Geometry: final body of the model. Coordinates: model frame, mm. Face numbers are marked on the shaded views. A direction names the side the tool comes from. Coordinates: 2 decimals unless noted, no trailing zeros. Write each loop counter-clockwise with the first axis right and the second up, starting at its lowest first coordinate (ties: lowest second). Pieces come first, ordered by that corner, then holes. Notation, with made-up numbers: (22.25, 61.25) - (44.25, 61.25) arc R10 ccw to (44.25, 79.25) - close; hole circle Ø9 at (23, -1). An arc over 180 degrees is marked (long way). Answer as a JSON object with one key per item and string values. Group by question number.
Item 1: First-contact query: pin 1 Ø1.5 at (x, z) = (72.5, 15) entering from -Y; pin 2 Ø8 at (x, z) = (72, 11.5) entering from -Y; pin 3 Ø11 at (x, y) = (62.5, 107) entering from +Z; pin 4 Ø9.5 at (x, y) = (67, 85.5) entering from +Z. Flat tips, straight axial feed; report the tip coordinate or a pass-through.
Item 2: Section B-B on x = 72.5. Return loops of the section in (y, z).
Item 3: Set-up query: the marked faces 4, 5, 6, 7 and 8. Return all of +Z, -Z, +X, -X, +Y, -Y with unobstructed straight access to the full face (end or side cutting, diameter ignored); none if empty.
Item 4: Section A-A on z = 4.25. Return loops of the section in (x, y).
Item 5: Section C-C on y = 12.5. Return loops of the section in (x, z), and give its area (3 significant figures).
Item 6: Line query: line 1 along Y through (x, z) = (55, 9); line 2 along Y through (x, z) = (58, 9.5); line 3 along Y through (x, z) = (78.5, 24). Output: solid intervals per line, ascending. Write a range as from..to.
Item 7: Section D-D on z = 21. Return loops of the section in (x, y), and give its area (3 significant figures).
Item 8: Mould query, pull axis X, two halves, no side actions, for the marked faces 1, 2 and 3. Classes: pulls with the +X half, pulls with the -X half, needs draft (parallel to the pull), parting line crosses it, or undercut.
```python
from build123d import *

# Parameters (mm, degrees)
F0_W     = 30
F0_H     = 57
F0_H_2   = 3
F0_H_3   = 22.2
F0_H_4   = 8.5
F1_DEPTH = 3
F2_DEPTH = 30
F3_DEPTH = 13
F4_DEPTH = 10
F5_W     = 20
F5_H     = 41
F6_DEPTH = 13


# Not quite as in the source:
# - a feature of the source that left no trace in its solid (it failed there, or was rolled back) is left out


with BuildPart() as f1:
    # F0 (on Top) → F1 (new body)
    with BuildSketch(Plane.XY):
        with Locations((67.8492219866, 28.5)):
            Rectangle(F0_W, F0_H)
        with Locations((67.8492219866, 58.5)):
            Rectangle(F0_W, F0_H_2)
        with Locations((67.8492219866, 71.1)):
            Rectangle(F0_W, F0_H_3)
        with Locations((67.8492219866, 86.45)):
            Rectangle(F0_W, F0_H_4)
        with Locations((67.8492219866, 101.8)):
            Rectangle(F0_W, F0_H_3)
        with Locations((67.8492219866, 114.4)):
            Rectangle(F0_W, F0_H_2)
    extrude(amount=F1_DEPTH)

    # F0 (on Top) → F2 (join)
    with BuildSketch(Plane.XY):
        with Locations((67.8492219866, 58.5)):
            Rectangle(F0_W, F0_H_2)
        with Locations((67.8492219866, 114.4)):
            Rectangle(F0_W, F0_H_2)
    extrude(amount=F2_DEPTH)

    # F0 (on Top) → F3 (join)
    with BuildSketch(Plane.XY):
        with Locations((67.8492219866, 86.45)):
            Rectangle(F0_W, F0_H_4)
    extrude(amount=F3_DEPTH)

    # F4 (add): a face of the model
    f4_faces = [f1.faces().sort_by_distance(p)[0] for p in [
        (67.8492219866, 28.5, 3),
    ]]
    extrude(f4_faces, amount=F4_DEPTH)

    # F5 (on face) → F6 (cut, through all)
    with BuildSketch(Plane.XY.offset(13)):
        with Locations((67.8492219866, 30.5)):
            Rectangle(F5_W, F5_H)
    extrude(amount=-F6_DEPTH, mode=Mode.SUBTRACT)


solid = f1.part
```
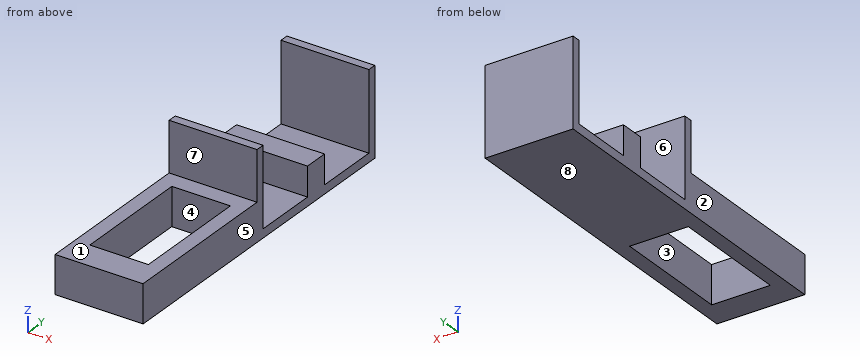
Checks:
{
 "1": {"pin 1": "y = 57", "pin 2": "y = 0", "pin 3": "z = 3", "pin 4": "z = 13"},
 "2": {"outline": "(0, 0) - (10, 0) - (10, 13) - (0, 13) - close; (51, 0) - (115.9, 0) - (115.9, 30) - (112.9, 30) - (112.9, 3) - (90.7, 3) - (90.7, 13) - (82.2, 13) - (82.2, 3) - (60, 3) - (60, 30) - (57, 30) - (57, 13) - (51, 13) - close"},
 "3": {"face 4": "+Z, -Z", "face 5": "+Z, -Z, +X, +Y, -Y", "face 6": "+Z, +X, -X", "face 7": "+Z, +X, -X, -Y", "face 8": "-Z, +X, -X, +Y, -Y"},
 "4": {"outline": "(52.85, 0) - (82.85, 0) - (82.85, 60) - (52.85, 60) - close; (52.85, 82.2) - (82.85, 82.2) - (82.85, 90.7) - (52.85, 90.7) - close; (52.85, 112.9) - (82.85, 112.9) - (82.85, 115.9) - (52.85, 115.9) - close; hole (57.85, 10) - (77.85, 10) - (77.85, 51) - (57.85, 51) - close"},
 "5": {"outline": "(52.85, 0) - (57.85, 0) - (57.85, 13) - (52.85, 13) - close; (77.85, 0) - (82.85, 0) - (82.85, 13) - (77.85, 13) - close", "area": "130 mm^2"},
 "6": {"line 1": "0..60, 82.2..90.7, 112.9..115.9", "line 2": "0..10, 51..60, 82.2..90.7, 112.9..115.9", "line 3": "57..60, 112.9..115.9"},
 "7": {"outline": "(52.85, 57) - (82.85, 57) - (82.85, 60) - (52.85, 60) - close; (52.85, 112.9) - (82.85, 112.9) - (82.85, 115.9) - (52.85, 115.9) - close", "area": "180 mm^2"},
 "8": {"face 1": "needs draft", "face 2": "pulls with the -X half", "face 3": "undercut"}
}
